Check sheet for the modelled part. Datum: model origin and axes. Units: mm. Face numbers are marked on the shaded views. A direction names the side the tool comes from. Give positions to 0.01 mm unless a question says otherwise; leave off trailing zeros. Write each loop counter-clockwise with the first axis right and the second up, starting at its lowest first coordinate (ties: lowest second). Pieces come first, ordered by that corner, then holes. Notation, with made-up numbers: M 12,46 L 67,46 A27 ccw 67,76 Z; hole C -10.75,27 d8. An arc over 180 degrees is marked long. Write item = value, one per line. Start each with the question number.
1) Draft check along X on the marked faces 1, 2 and 3. Enter one of: pulls with the +X half, pulls with the -X half, needs draft (parallel to the pull), parting line crosses it, or undercut.
2) Gauge pin test, flat ends, axial feed: pin 1 (8 mm diameter, centred on y = -10, z = -8, fed in from +X); pin 2 (8 mm diameter, centred on x = -7, y = 10, fed in from -Z); pin 3 (4 mm diameter, centred on x = -12.5, z = -5, fed in from -Y); pin 4 (1.5 mm diameter, centred on y = 14.5, z = -2.5, fed in from -X). Record the tip position at first contact, or that the pin passes through.
3) Sectioned sample at D-D, the plane x = -0.5. Record the cut outline in (y, z).
4) Sectioned sample at A-A, the plane y = -6. Record the cut outline in (x, z).
5) Scan lines: L1, parallel to Y at x = 8, z = 1.35; L2, parallel to Y at x = 5.5, z = -3; L3, parallel to Y at x = -5, z = -14.5. Record each from-to range of solid material in increasing order.
6) Sectioned sample at C-C, the plane y = 7. Record the cut outline in (x, z).
7) Set-up check for the marked faces 4, 5 and 6: record each of +Z, -Z, +X, -X, +Y, -Y from which the full face is reachable in a straight line by a thin tool's end or side.
8) Sectioned sample at B-B, the plane x = -14. Record the cut outline in (y, z), then the cut area to 3 significant figures.
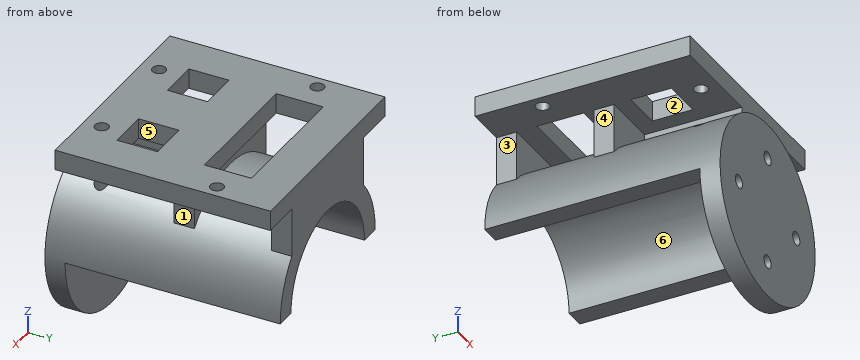
from build123d import *

# Parameters (mm, degrees)
SKETCH1_W                = 32
SKETCH1_H                = 32
SKETCH1_R                = 1
SKETCH1_W_2              = 20
SKETCH1_H_2              = 7
SKETCH1_W_3              = 6
SKETCH1_H_3              = 6
BOSS_EXTRUDE1_DEPTH      = 3
SKETCH2_R                = 13.25
SKETCH2_R_2              = 1
BOSS_EXTRUDE2_DEPTH      = 3
BOSS_EXTRUDE3_DEPTH      = 32
BOSS_EXTRUDE4_REACH      = 40.374
BOSS_EXTRUDE4_END_RADIUS = 13.25
SKETCH4_W                = 20
SKETCH4_H                = 3
SKETCH6_R                = 1
CUT_EXTRUDE1_DEPTH       = 41.707032562


with BuildPart() as part:
    # Sketch1 → Boss-Extrude1 (new body)
    with BuildSketch(Plane.XY):
        Rectangle(SKETCH1_W, SKETCH1_H)
        with Locations((14, 7)):
            Circle(SKETCH1_R, mode=Mode.SUBTRACT)
        with Locations(Location((-14, 7, 0), (0, 0, 180))):
            Circle(SKETCH1_R, mode=Mode.SUBTRACT)
        with Locations((-8, -13.347936253)):
            Circle(SKETCH1_R, mode=Mode.SUBTRACT)
        with Locations(Location((8, -13.347936253, 0), (0, 0, 180))):
            Circle(SKETCH1_R, mode=Mode.SUBTRACT)
        with Locations((0, 6.5)):
            Rectangle(SKETCH1_W_2, SKETCH1_H_2, mode=Mode.SUBTRACT)
        with Locations((-7, -7)):
            Rectangle(SKETCH1_W_3, SKETCH1_H_3, mode=Mode.SUBTRACT)
        with Locations((7, -7)):
            Rectangle(SKETCH1_W_3, SKETCH1_H_3, mode=Mode.SUBTRACT)
    extrude(amount=BOSS_EXTRUDE1_DEPTH)



with BuildPart() as body_2:
    # Sketch2 → Boss-Extrude2 (new body)
    with BuildSketch(Plane.XZ.offset(16)):
        with Locations(Location((0, -16, 0), (0, 0, 270))):
            Circle(SKETCH2_R)
        with Locations(Location((-8, -16, 0), (0, 0, 270))):
            Circle(SKETCH2_R_2, mode=Mode.SUBTRACT)
        with Locations(Location((0, -8, 0), (0, 0, 270))):
            Circle(SKETCH2_R_2, mode=Mode.SUBTRACT)
        with Locations(Location((8, -16, 0), (0, 0, 270))):
            Circle(SKETCH2_R_2, mode=Mode.SUBTRACT)
        with Locations(Location((0, -24, 0), (0, 0, 270))):
            Circle(SKETCH2_R_2, mode=Mode.SUBTRACT)
    extrude(amount=BOSS_EXTRUDE2_DEPTH)

    # Sketch3 → Boss-Extrude3 (add)
    with BuildSketch(Plane(origin=(0, -16, 0), x_dir=(1, 0, 0), z_dir=(0, 1, 0))):
        with BuildLine():
            Line((-13.25, 16), (-10.25, 16))
            ThreePointArc((-10.25, 16), (0, 5.75), (10.25, 16))
            Line((10.25, 16), (13.25, 16))
            ThreePointArc((13.25, 16), (0, 2.75), (-13.25, 16))
        make_face()
    extrude(amount=BOSS_EXTRUDE3_DEPTH)


with BuildPart() as part_1:
    add(part.part)

    add(body_2.part)  # Boss-Extrude4 merges body 2
    # Boss-Extrude4: up to this cylinder (the profile starts outside it)
    boss_extrude4_end = Plane(origin=(0, 5.411232, -16), z_dir=(0, 1, 0)) * Cylinder(BOSS_EXTRUDE4_END_RADIUS, 126.425536, mode=Mode.PRIVATE)
    # Sketch4 → Boss-Extrude4 (add, up to the surface)
    with BuildSketch(Plane(origin=(0, 0, 0), x_dir=(-1, 0, 0), z_dir=(0, 0, -1)), mode=Mode.PRIVATE) as boss_extrude4_sk1:
        with Locations((0, 14.5)):
            Rectangle(SKETCH4_W, SKETCH4_H)
    boss_extrude4_tool1 = extrude(boss_extrude4_sk1.sketch, amount=BOSS_EXTRUDE4_REACH, mode=Mode.PRIVATE) - boss_extrude4_end
    add(boss_extrude4_tool1.solids().sort_by_distance((0, 14.5, 0))[0])
    # Sketch4 → Boss-Extrude4 (add, up to the surface)
    with BuildSketch(Plane(origin=(0, 0, 0), x_dir=(-1, 0, 0), z_dir=(0, 0, -1)), mode=Mode.PRIVATE) as boss_extrude4_sk2:
        Polygon((10, 1.5), (-10, 1.5), (-10, -1.5), (-1.5, -1.5), (-1.5, -16), (1.5, -16), (1.5, -1.5), (10, -1.5), align=None)
    boss_extrude4_tool2 = extrude(boss_extrude4_sk2.sketch, amount=BOSS_EXTRUDE4_REACH, mode=Mode.PRIVATE) - boss_extrude4_end
    add(boss_extrude4_tool2.solids().sort_by_distance((0, -3.677536, 0))[0])

    # Sketch6 → Cut-Extrude1 (cut, through all)
    with BuildSketch(Plane.XY.offset(3)):
        with Locations(Location((8, -13.347936253, 0), (0, 0, 180))):
            Circle(SKETCH6_R)
        with Locations((-8, -13.347936253)):
            Circle(SKETCH6_R)
    extrude(amount=-CUT_EXTRUDE1_DEPTH, mode=Mode.SUBTRACT)


solid = part_1.part
Data:
q1.face_1 = pulls with the +X half
q1.face_2 = undercut
q1.face_3 = pulls with the -X half
q2.pin_1 = 12.63
q2.pin_2 = -16
q2.pin_3 = through
q2.pin_4 = -10
q3.outline = M -19,-29.24 L -16,-29.24 L -16,-24.87 L -19,-24.87 Z; M -19,-23.13 L -16,-23.13 L -16,-8.87 L -19,-8.87 Z; M -19,-7.13 L -16,-7.13 L -16,-5.76 L 16,-5.76 L 16,3 L 10,3 L 10,0 L 13,0 L 13,-2.76 L 1.5,-2.76 L 1.5,0 L 3,0 L 3,3 L -16,3 L -16,-2.76 L -19,-2.76 Z
q4.outline = M -16,0 L -10,0 L -10,3 L -16,3 Z; M -13.25,-16 L -10.25,-16 A10.25 cw 10.25,-16 L 13.25,-16 A13.25 ccw 1.5,-2.84 L 1.5,0 L 4,0 L 4,3 L -4,3 L -4,0 L -1.5,0 L -1.5,-2.84 A13.25 ccw Z; M 10,0 L 16,0 L 16,3 L 10,3 Z
q5.L1 = -16 to -14.35, -12.35 to -10, -4 to 3, 10 to 16
q5.L2 = -1.5 to 1.5, 13 to 16
q5.L3 = -19 to -16
q6.outline = M -16,0 L -15,0 L -15,3 L -16,3 Z; M -13.25,-16 L -10.25,-16 A10.25 cw 10.25,-16 L 13.25,-16 A13.25 ccw Z; M -13,0 L -10,0 L -10,3 L -13,3 Z; M 10,0 L 13,0 L 13,3 L 10,3 Z; M 15,0 L 16,0 L 16,3 L 15,3 Z
q7.face_4 = -X, +Y, -Y
q7.face_5 = +Z
q7.face_6 = -Z, +Y
q8.outline = M -16,0 L 6,0 L 6,3 L -16,3 Z; M 8,0 L 16,0 L 16,3 L 8,3 Z
q8.area = 90.0 mm2
